from build123d import *

# Parameters (mm, degrees)
F0_R     = 11.303
F1_DEPTH = 7.0104


# Not quite as in the source:
# - a feature names something its author has since deleted; it is built from what else it names


with BuildPart() as f1:
    # F0 (on Top) → F1 (new body)
    with BuildSketch(Plane.XY):
        with BuildLine():
            ThreePointArc((-8.4576062893, 17.6302414744), (0, 14.605), (8.4576062893, 17.6302414744))
            ThreePointArc((8.4576062893, 17.6302414744), (12.0541363205, 22.2373670497), (13.335, 27.94))
            ThreePointArc((13.335, 27.94), (9.9631286308, 36.8033116207), (1.552728851, 41.1842915294))
            ThreePointArc((1.552728851, 41.1842915294), (0, 41.2234534857), (-1.552728851, 41.1842915294))
            ThreePointArc((-1.552728851, 41.1842915294), (-12.7964847088, 31.6912936565), (-8.4576062893, 17.6302414744))
        make_face()
        with Locations((0, 27.94)):
            Circle(F0_R, mode=Mode.SUBTRACT)
        with BuildLine():
            ThreePointArc((-8.4410840797, 11.1314419353), (0, 13.97), (8.4410840797, 11.1314419353))
            ThreePointArc((8.4410840797, 11.1314419353), (7.023943937, 14.3844655708), (8.4576062893, 17.6302414744))
            ThreePointArc((8.4576062893, 17.6302414744), (0, 14.605), (-8.4576062893, 17.6302414744))
            ThreePointArc((-8.4576062893, 17.6302414744), (-7.1686601212, 14.3840976519), (-8.4410840797, 11.1314419353))
        make_face()
        with BuildLine():
            ThreePointArc((8.4410840797, -11.1314419353), (12.5116514616, -6.2144571527), (13.97, 0))
            ThreePointArc((13.97, 0), (12.5116514616, 6.2144571527), (8.4410840797, 11.1314419353))
            ThreePointArc((8.4410840797, 11.1314419353), (0, 13.97), (-8.4410840797, 11.1314419353))
            ThreePointArc((-8.4410840797, 11.1314419353), (-12.5116514616, 6.2144571527), (-13.97, 0))
            ThreePointArc((-13.97, 0), (-12.5116514616, -6.2144571527), (-8.4410840797, -11.1314419353))
            ThreePointArc((-8.4410840797, -11.1314419353), (0, -13.97), (8.4410840797, -11.1314419353))
        make_face()
        Circle(F0_R, mode=Mode.SUBTRACT)
        with BuildLine():
            ThreePointArc((8.4410840797, -17.616709606), (7.0831122532, -14.3740757706), (8.4410840797, -11.1314419353))
            ThreePointArc((8.4410840797, -11.1314419353), (0, -13.97), (-8.4410840797, -11.1314419353))
            ThreePointArc((-8.4410840797, -11.1314419353), (-7.1012049909, -14.3740757706), (-8.4410840797, -17.616709606))
            ThreePointArc((-8.4410840797, -17.616709606), (0, -14.605), (8.4410840797, -17.616709606))
        make_face()
        with BuildLine():
            ThreePointArc((13.335, -27.94), (12.0495659922, -22.2277163587), (8.4410840797, -17.616709606))
            ThreePointArc((8.4410840797, -17.616709606), (0, -14.605), (-8.4410840797, -17.616709606))
            ThreePointArc((-8.4410840797, -17.616709606), (-12.9933407259, -30.9392201953), (-3.0623665698, -40.9186030062))
            ThreePointArc((-3.0623665698, -40.9186030062), (-0.2065651455, -41.0979009929), (2.6534571531, -41.0083354004))
            ThreePointArc((2.6534571531, -41.0083354004), (10.3248747241, -36.3791461021), (13.335, -27.94))
        make_face()
        with Locations((0, -27.94)):
            Circle(F0_R, mode=Mode.SUBTRACT)
        with BuildLine():
            ThreePointArc((-13.97, 0), (-12.5116514616, 6.2144571527), (-8.4410840797, 11.1314419353))
            ThreePointArc((-8.4410840797, 11.1314419353), (-7.1686601212, 14.3840976519), (-8.4576062893, 17.6302414744))
            ThreePointArc((-8.4576062893, 17.6302414744), (-12.7964847088, 31.6912936565), (-1.552728851, 41.1842915294))
            ThreePointArc((-1.552728851, 41.1842915294), (-15.6144282797, 36.9723347017), (-26.1298660189, 26.7303846776))
            Line((-26.1298660189, 26.7303846776), (-13.97, 0))
        make_face()
        with BuildLine():
            ThreePointArc((8.4410840797, 11.1314419353), (12.5116514616, 6.2144571527), (13.97, 0))
            Line((13.97, 0), (26.1298660189, 26.7303846776))
            ThreePointArc((26.1298660189, 26.7303846776), (15.6144282797, 36.9723347017), (1.552728851, 41.1842915294))
            ThreePointArc((1.552728851, 41.1842915294), (9.9631286308, 36.8033116207), (13.335, 27.94))
            ThreePointArc((13.335, 27.94), (12.0541363205, 22.2373670497), (8.4576062893, 17.6302414744))
            ThreePointArc((8.4576062893, 17.6302414744), (7.023943937, 14.3844655708), (8.4410840797, 11.1314419353))
        make_face()
        with BuildLine():
            Line((26.1298660189, -26.7303846776), (13.97, 0))
            ThreePointArc((13.97, 0), (12.5116514616, -6.2144571527), (8.4410840797, -11.1314419353))
            ThreePointArc((8.4410840797, -11.1314419353), (7.0831122532, -14.3740757706), (8.4410840797, -17.616709606))
            ThreePointArc((8.4410840797, -17.616709606), (12.0495659922, -22.2277163587), (13.335, -27.94))
            ThreePointArc((13.335, -27.94), (10.3248747241, -36.3791461021), (2.6534571531, -41.0083354004))
            ThreePointArc((2.6534571531, -41.0083354004), (16.0937498742, -36.6680054018), (26.1298660189, -26.7303846776))
        make_face()
        with BuildLine():
            ThreePointArc((-8.4410840797, -17.616709606), (-7.1012049909, -14.3740757706), (-8.4410840797, -11.1314419353))
            ThreePointArc((-8.4410840797, -11.1314419353), (-12.5116514616, -6.2144571527), (-13.97, 0))
            Line((-13.97, 0), (-25.8976111474, -26.2198311856))
            ThreePointArc((-25.8976111474, -26.2198311856), (-16.209405425, -36.2559483923), (-3.0623665698, -40.9186030062))
            ThreePointArc((-3.0623665698, -40.9186030062), (-12.9933407259, -30.9392201953), (-8.4410840797, -17.616709606))
        make_face()
    extrude(amount=F1_DEPTH)


solid = f1.part
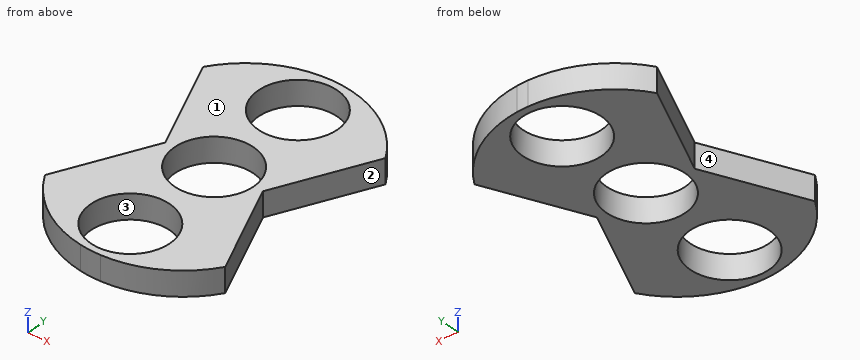
Geometry: final body of the model. Coordinates: model frame, mm. Face numbers are marked on the shaded views. Round coordinates to 2 decimals unless told otherwise and drop trailing zeros. Loops run counter-clockwise (first coordinate to the right, second up) from the corner with the lowest first, then second, coordinate; pieces in that order, holes last. Notation, with made-up numbers: (61, 42) -> (103, 42) arc R18 cw to (103, 63) -> close; hole circle Ø5 at (-35.5, 2). An arc over 180 degrees is marked (long way). One line per question, with ' | ' between items. Start each with the question number.
1. Section D-D on y = -27.94. Output: boundary loops of the cut face in (x, z), and give its area (3 significant figures).
2. Section B-B on y = -3.5. Output: boundary loops of the cut face in (x, z).
3. Mould query, pull axis X, two halves, no side actions, for the marked faces 1, 2, 3 and 4. Classes: pulls with the +X half, pulls with the -X half, needs draft (parallel to the pull), parting line crosses it, or undercut.
4. Contact query for flat-ended pins moving along their axis: pin 1 (4 mm diameter, centred on x = 8.5, z = 3, fed in from -Y); pin 2 (1.5 mm diameter, centred on y = -2.5, z = 1, fed in from -X); pin 3 (4 mm diameter, centred on y = -5.5, z = 1.5, fed in from +X); pin 4 (13.5 mm diameter, centred on x = 0, y = 27.94, fed in from +Z). Output: stop coordinate, or through.
5. Section A-A on z = 5.25. Output: boundary loops of the cut face in (x, y), and give its area (3 significant figures).
6. Line query: line 1 along Y through (x, z) = (0, 3.5); line 2 along Y through (x, z) = (-3, 6); line 3 along X through (y, z) = (8.5, 6). Output: solid intervals per line, ascending. Write a range as [from, to].
7. Section C-C on x = 0. Output: boundary loops of the cut face in (y, z).
Returned:
1) outline: (-24.79, 0) -> (-11.3, 0) -> (-11.3, 7.01) -> (-24.79, 7.01) -> close; (11.3, 0) -> (25.34, 0) -> (25.34, 7.01) -> (11.3, 7.01) -> close | area: 193 mm2
2) outline: (-15.56, 0) -> (-10.75, 0) -> (-10.75, 7.01) -> (-15.56, 7.01) -> close; (10.75, 0) -> (15.56, 0) -> (15.56, 7.01) -> (10.75, 7.01) -> close
3) face 1: needs draft | face 2: pulls with the +X half | face 3: undercut | face 4: pulls with the -X half
4) pin 1: stops at y = -40.46 | pin 2: stops at x = -15.45 | pin 3: stops at x = 17.38 | pin 4: passes through
5) outline: (-26.13, 26.73) -> (-13.97, 0) -> (-25.9, -26.22) arc R30.45 ccw to (26.13, -26.73) -> (13.97, 0) -> (26.13, 26.73) arc R30.8 ccw to start; hole circle Ø22.61 at (0, -27.94); hole circle Ø22.61 at (0, 0); hole circle Ø22.61 at (0, 27.94) | area: 2,000 mm2
6) line 1: y = [-41.1, -39.24], [-16.64, -11.3], [11.3, 16.64], [39.24, 41.22] | line 2: y = [-40.93, -38.84], [-17.04, -10.9], [10.9, 17.04], [38.84, 41.08] | line 3: x = [-17.84, -7.45], [7.45, 17.84]
7) outline: (-41.1, 0) -> (-39.24, 0) -> (-39.24, 7.01) -> (-41.1, 7.01) -> close; (-16.64, 0) -> (-11.3, 0) -> (-11.3, 7.01) -> (-16.64, 7.01) -> close; (11.3, 0) -> (16.64, 0) -> (16.64, 7.01) -> (11.3, 7.01) -> close; (39.24, 0) -> (41.22, 0) -> (41.22, 7.01) -> (39.24, 7.01) -> close
